Job drawing, mm, ordinate dimensions from the low corner. One solid piece. A direction names the side the tool comes from. Give positions to 0.01 mm unless a question says otherwise; leave off trailing zeros. Loops run counter-clockwise (first coordinate to the right, second up) from the corner with the lowest first, then second, coordinate; pieces in that order, holes last. Notation, with made-up numbers: M 7.5,15.5 L 23.5,15.5 A14 ccw 23.5,28.5 Z; hole C -8,71.25 d4. An arc over 180 degrees is marked long. Answer as CSV lines item,"result".
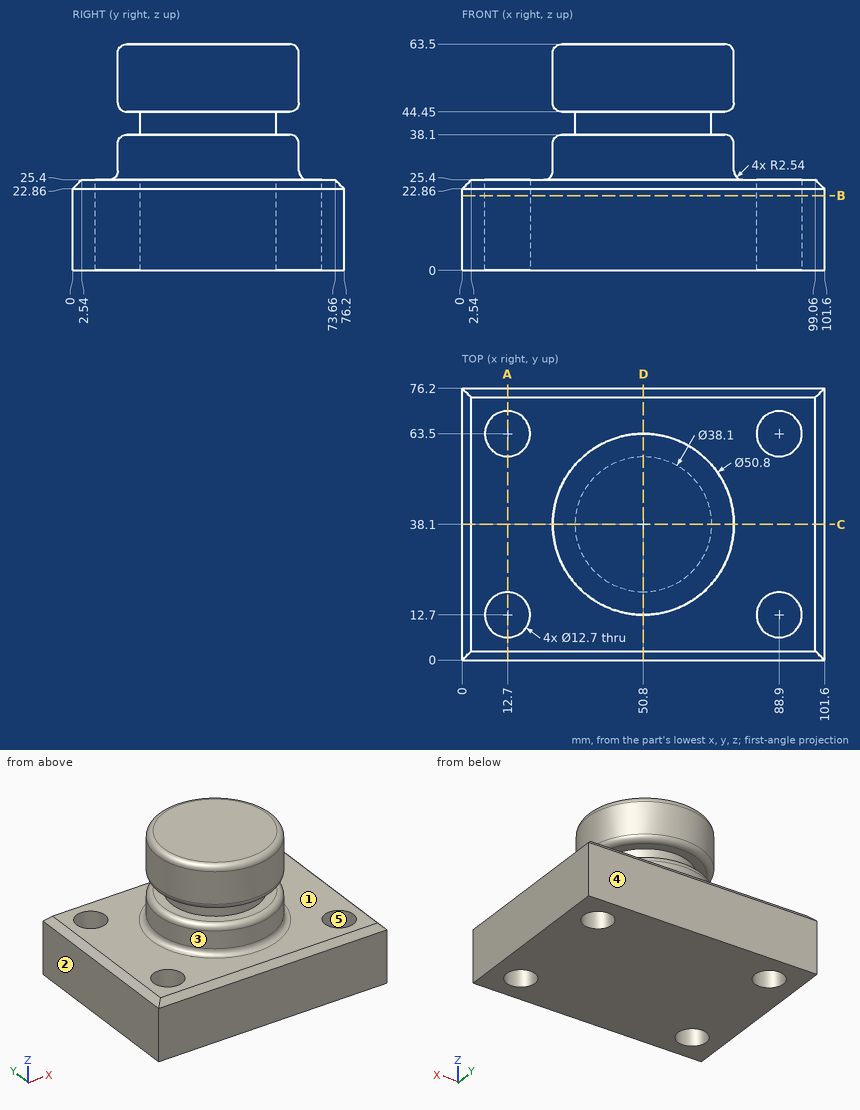
1) Band-saw the part on B-B on z = 21. Give the cut face in (x, y), and give its area (3 significant figures).
Answer below:
outline,"M 0,0 L 101.6,0 L 101.6,76.2 L 0,76.2 Z; hole C 12.7,12.7 d12.7; hole C 12.7,63.5 d12.7; hole C 88.9,12.7 d12.7; hole C 88.9,63.5 d12.7"
area,"7,240 mm^2"
2) Drill centre lines: line 1 (Y direction, x = 12.7, z = 17.5); line 2 (Z direction, x = 30.5, y = 35); line 3 (X direction, y = 17, z = 8.5). Where is each one in solid material? Low to high. Write a range as from..to.
Answer below:
line 1,"y = 0..6.35, 19.05..57.15, 69.85..76.2"
line 2,"z = 0..38.1, 44.45..63.5"
line 3,"x = 0..8.03, 17.37..84.23, 93.57..101.6"
3) Mould opens along X. For the marked faces 3, 4 and 5 say: +X half, -X half, draft (parallel to the pull), parting line (faces both ways), or undercut.
Answer below:
face 3,"parting line"
face 4,"draft"
face 5,"undercut"
4) Band-saw the part on C-C on y = 38.1. Give the cut face in (x, z).
Answer below:
outline,"M 0,0 L 101.6,0 L 101.6,22.86 L 99.06,25.4 L 78.74,25.4 A2.54 cw 76.2,27.94 L 76.2,35.56 A2.54 ccw 73.66,38.1 L 69.85,38.1 L 69.85,44.45 L 73.66,44.45 A2.54 ccw 76.2,46.99 L 76.2,60.96 A2.54 ccw 73.66,63.5 L 27.94,63.5 A2.54 ccw 25.4,60.96 L 25.4,46.99 A2.54 ccw 27.94,44.45 L 31.75,44.45 L 31.75,38.1 L 27.94,38.1 A2.54 ccw 25.4,35.56 L 25.4,27.94 A2.54 cw 22.86,25.4 L 2.54,25.4 L 0,22.86 Z"
5) Flat gauge pins, fed straight in: pin 1 (1 mm diameter, centred on y = 35, z = 33, fed in from +X); pin 2 (23 mm diameter, centred on x = 58, y = 41, fed in from -Z); pin 3 (14.5 mm diameter, centred on x = 88.9, y = 12.7, fed in from +Z); pin 4 (8 mm diameter, centred on y = 64.5, z = 35, fed in from +X) (3 decimals). Where does each tip first touch, or does it go through?
Answer below:
pin 1,"stops at x = 76.07"
pin 2,"stops at z = 0"
pin 3,"stops at z = 25.4"
pin 4,"stops at x = 62.775"
6) Band-saw the part on D-D on x = 50.8. Give the cut face in (y, z), and give its area (3 significant figures).
Answer below:
outline,"M 0,0 L 76.2,0 L 76.2,22.86 L 73.66,25.4 L 66.04,25.4 A2.54 cw 63.5,27.94 L 63.5,35.56 A2.54 ccw 60.96,38.1 L 57.15,38.1 L 57.15,44.45 L 60.96,44.45 A2.54 ccw 63.5,46.99 L 63.5,60.96 A2.54 ccw 60.96,63.5 L 15.24,63.5 A2.54 ccw 12.7,60.96 L 12.7,46.99 A2.54 ccw 15.24,44.45 L 19.05,44.45 L 19.05,38.1 L 15.24,38.1 A2.54 ccw 12.7,35.56 L 12.7,27.94 A2.54 cw 10.16,25.4 L 2.54,25.4 L 0,22.86 Z"
area,"3,780 mm^2"
7) Band-saw the part on A-A on x = 12.7. Give the cut face in (y, z), and give its area (3 significant figures).
Answer below:
outline,"M 0,0 L 6.35,0 L 6.35,25.4 L 2.54,25.4 L 0,22.86 Z; M 19.05,0 L 57.15,0 L 57.15,25.4 L 19.05,25.4 Z; M 69.85,0 L 76.2,0 L 76.2,22.86 L 73.66,25.4 L 69.85,25.4 Z"
area,"1,280 mm^2"
8) Which spindle directions (+Z, -Z, +X, -X, +Y, -Y) get a long thin tool onto all of the face, cutting with end or side? Do the marked faces 1 and 2. Say none if no direction does.
Answer below:
face 1,"+Z"
face 2,"+Z, -Z, -X, +Y, -Y"
